from build123d import *

# Parameters (mm, degrees)
EXTRUDE_1_DEPTH     = 10
CUT_EXTRUDE_2_DEPTH = 8


with BuildPart() as part:
    # 草图1 → 凸台-拉伸1 (new body)
    with BuildSketch(Plane.XY):
        with BuildLine():
            Line((-10, 24.791076412), (-15.93770494, 3.262397709))
            ThreePointArc((-15.93770494, 3.262397709), (0, -12.675307231), (15.93770494, 3.262397709))
            Line((15.93770494, 3.262397709), (10, 24.791076412))
            ThreePointArc((10, 24.791076412), (0, 34.791076412), (-10, 24.791076412))
        make_face()
    extrude(amount=-EXTRUDE_1_DEPTH)

    # 草图3 → 切除-拉伸2 (cut)
    with BuildSketch(Plane.XY):
        with BuildLine():
            Line((0, 23.501027712), (-0.472402553, 21.711669494))
            ThreePointArc((-0.472402553, 21.711669494), (-0.489109338, 21.709069686), (-0.50580182, 21.70637957))
            Line((-0.50580182, 21.70637957), (-1.508025445, 23.262179946))
            Line((-1.508025445, 23.262179946), (-1.404364874, 21.414418736))
            ThreePointArc((-1.404364874, 21.414418736), (-1.419450586, 21.40678349), (-1.434494788, 21.399066778))
            Line((-1.434494788, 21.399066778), (-2.868434853, 22.569016731))
            Line((-2.868434853, 22.569016731), (-2.198858175, 20.84372427))
            ThreePointArc((-2.198858175, 20.84372427), (-2.210846119, 20.831800979), (-2.22276941, 20.819813035))
            Line((-2.22276941, 20.819813035), (-3.948061872, 21.489389712))
            Line((-3.948061872, 21.489389712), (-2.778111918, 20.055449647))
            ThreePointArc((-2.778111918, 20.055449647), (-2.785828631, 20.040405445), (-2.793463876, 20.025319733))
            Line((-2.793463876, 20.025319733), (-4.641225087, 20.128980305))
            Line((-4.641225087, 20.128980305), (-3.085424711, 19.12675668))
            ThreePointArc((-3.085424711, 19.12675668), (-3.088114827, 19.110064198), (-3.090714635, 19.093357413))
            Line((-3.090714635, 19.093357413), (-4.880072853, 18.620954859))
            Line((-4.880072853, 18.620954859), (-3.090714635, 18.148552306))
            ThreePointArc((-3.090714635, 18.148552306), (-3.088114827, 18.131845521), (-3.085424711, 18.115153039))
            Line((-3.085424711, 18.115153039), (-4.641225087, 17.112929414))
            Line((-4.641225087, 17.112929414), (-2.793463876, 17.216589986))
            ThreePointArc((-2.793463876, 17.216589986), (-2.785828631, 17.201504274), (-2.778111918, 17.186460072))
            Line((-2.778111918, 17.186460072), (-3.948061872, 15.752520006))
            Line((-3.948061872, 15.752520006), (-2.22276941, 16.422096684))
            ThreePointArc((-2.22276941, 16.422096684), (-2.210846119, 16.41010874), (-2.198858175, 16.398185449))
            Line((-2.198858175, 16.398185449), (-2.868434853, 14.672892987))
            Line((-2.868434853, 14.672892987), (-1.434494788, 15.842842941))
            ThreePointArc((-1.434494788, 15.842842941), (-1.419450586, 15.835126228), (-1.404364874, 15.827490983))
            Line((-1.404364874, 15.827490983), (-1.508025445, 13.979729772))
            Line((-1.508025445, 13.979729772), (-0.50580182, 15.535530148))
            ThreePointArc((-0.50580182, 15.535530148), (-0.489109338, 15.532840033), (-0.472402553, 15.530240224))
            Line((-0.472402553, 15.530240224), (0, 13.740882006))
            Line((0, 13.740882006), (0.472402553, 15.530240224))
            ThreePointArc((0.472402553, 15.530240224), (0.489109338, 15.532840033), (0.50580182, 15.535530148))
            Line((0.50580182, 15.535530148), (1.508025445, 13.979729772))
            Line((1.508025445, 13.979729772), (1.404364874, 15.827490983))
            ThreePointArc((1.404364874, 15.827490983), (1.419450586, 15.835126228), (1.434494788, 15.842842941))
            Line((1.434494788, 15.842842941), (2.868434853, 14.672892987))
            Line((2.868434853, 14.672892987), (2.198858175, 16.398185449))
            ThreePointArc((2.198858175, 16.398185449), (2.210846119, 16.41010874), (2.22276941, 16.422096684))
            Line((2.22276941, 16.422096684), (3.948061872, 15.752520006))
            Line((3.948061872, 15.752520006), (2.778111918, 17.186460072))
            ThreePointArc((2.778111918, 17.186460072), (2.785828631, 17.201504274), (2.793463876, 17.216589986))
            Line((2.793463876, 17.216589986), (4.641225087, 17.112929414))
            Line((4.641225087, 17.112929414), (3.085424711, 18.115153039))
            ThreePointArc((3.085424711, 18.115153039), (3.088114827, 18.131845521), (3.090714635, 18.148552306))
            Line((3.090714635, 18.148552306), (4.880072853, 18.620954859))
            Line((4.880072853, 18.620954859), (3.090714635, 19.093357413))
            ThreePointArc((3.090714635, 19.093357413), (3.088114827, 19.110064198), (3.085424711, 19.12675668))
            Line((3.085424711, 19.12675668), (4.641225087, 20.128980305))
            Line((4.641225087, 20.128980305), (2.793463876, 20.025319733))
            ThreePointArc((2.793463876, 20.025319733), (2.785828631, 20.040405445), (2.778111918, 20.055449647))
            Line((2.778111918, 20.055449647), (3.948061872, 21.489389712))
            Line((3.948061872, 21.489389712), (2.22276941, 20.819813035))
            ThreePointArc((2.22276941, 20.819813035), (2.210846119, 20.831800979), (2.198858175, 20.84372427))
            Line((2.198858175, 20.84372427), (2.868434853, 22.569016731))
            Line((2.868434853, 22.569016731), (1.434494788, 21.399066778))
            ThreePointArc((1.434494788, 21.399066778), (1.419450586, 21.40678349), (1.404364874, 21.414418736))
            Line((1.404364874, 21.414418736), (1.508025445, 23.262179946))
            Line((1.508025445, 23.262179946), (0.50580182, 21.70637957))
            ThreePointArc((0.50580182, 21.70637957), (0.489109338, 21.709069686), (0.472402553, 21.711669494))
            Line((0.472402553, 21.711669494), (0, 23.501027712))
        make_face()
    extrude(amount=-CUT_EXTRUDE_2_DEPTH, mode=Mode.SUBTRACT)


solid = part.part
Here's how the part is built. I have some questions about the finished solid (model axes, mm). Coordinates: 2 decimals unless noted, no trailing zeros. Write each loop counter-clockwise with the first axis right and the second up, starting at its lowest first coordinate (ties: lowest second). Pieces come first, ordered by that corner, then holes.
Item 1: I want a section at B-B on x = -6.5. Write out the boundary of the cut face in (y, z), and give its area (3 significant figures).
Item 2: If we mould it in two halves opening along Y, with no side actions, what happens to faces 1 (the flat face through (13.01, 13.88, -4.93)), 2 (the flat face through (-2.54, 21.72, -3.94)), 3 (the cylindrical face through (-0.35, -12.67, -4.93))? For each: +Y half, -Y half, draft (parallel to the pull), parting line (faces both ways), or undercut.
Item 3: Will these pins go through, and if not, where does the flat tip stop? pin 1 (5 mm diameter, centred on y = 5.5, z = -8, fed in from -X); pin 2 (3 mm diameter, centred on x = 5.5, z = -1.5, fed in from -Y); pin 3 (4 mm diameter, centred on x = -12.5, z = -7, fed in from -Y); pin 4 (1 mm diameter, centred on y = -2.5, z = -2, fed in from +X).
Item 4: If I drill on line 1 (Y direction, x = -3, z = -2.75) (1 decimal); line 2 (Y direction, x = 0, z = -8.75); line 3 (X direction, y = 19.5, z = -4.5), over which ranges is the centre line in solid material (lowest first)?
Item 5: I want a section at A-A on y = -2. Write out the boundary of the cut face in (x, z).
Findings below:
1. outline: (-11.29, -10) - (32.39, -10) - (32.39, 0) - (-11.29, 0) - close
1. area: 437 mm2
2. face 1: +Y half
2. face 2: undercut
2. face 3: -Y half
3. pin 1: stops at x = -15.94
3. pin 2: stops at y = -12.17
3. pin 3: stops at y = -8.73
3. pin 4: stops at x = 15.04
4. line 1: y = -12.4 to 16.1, 16.9 to 17.2, 20 to 20.3, 21.1 to 34.3
4. line 2: y = -12.68 to 34.79
4. line 3: x = -11.46 to -3.66, 3.66 to 11.46
5. outline: (-15.04, -10) - (15.04, -10) - (15.04, 0) - (-15.04, 0) - close
